For this review, take the finished solid that the model builds, in its own axes (mm). A direction names the side the tool comes from. Give positions to 0.01 mm unless a question says otherwise; leave off trailing zeros. Write each loop counter-clockwise with the first axis right and the second up, starting at its lowest first coordinate (ties: lowest second). Pieces come first, ordered by that corner, then holes. Notation, with made-up numbers: (-11, 43.25) -> (11, 43.25) arc R25 ccw to (11, 62.25) -> close; hole circle Ø9 at (24.25, 6.25). An arc over 180 degrees is marked (long way). Return JSON: item names as keys, results as strings.
from build123d import *

# Parameters (mm, degrees)
CROQUIS1_W               = 40.7
CROQUIS1_H               = 38
SALIENTE_EXTRUIR1_DEPTH  = 10.25
CROQUIS2_W               = 7
CROQUIS2_H               = 2.4
SALIENTE_EXTRUIR2_DEPTH  = 18.5
SALIENTE_EXTRUIR3_DEPTH  = 0.5
CORTAR_EXTRUIR1_DEPTH    = 2.4
SALIENTE_EXTRUIR4_DEPTH  = 2
CORTAR_EXTRUIR3_START    = -18.5
CORTAR_EXTRUIR3_DEPTH    = 18.5
CROQUIS10_R              = 7
SALIENTE_EXTRUIR5_DEPTH  = 0.75
CROQUIS11_R              = 5.5
SALIENTE_EXTRUIR6_DEPTH  = 1
CROQUIS12_R              = 3
SALIENTE_EXTRUIR7_DEPTH  = 5
CHAFL_N2_SIZE            = 0.5
CHAFL_N2_OF_MIRROR1_SIZE = 0.5


with BuildPart() as part:
    # Croquis1 → Saliente-Extruir1 (new body, symmetric)
    with BuildSketch(Plane.XY):
        Rectangle(CROQUIS1_W, CROQUIS1_H)
    extrude(amount=SALIENTE_EXTRUIR1_DEPTH, both=True)

    # Croquis2 → Saliente-Extruir2 (add)
    with BuildSketch(Plane.XY.offset(9.25)):
        with Locations((-23.85, 10.2)):
            Rectangle(CROQUIS2_W, CROQUIS2_H)
        with Locations((23.85, 10.2)):
            Rectangle(CROQUIS2_W, CROQUIS2_H)
    extrude(amount=-SALIENTE_EXTRUIR2_DEPTH)

    # Croquis3 → Saliente-Extruir3 (add, symmetric)
    with BuildSketch(Plane.XY):
        Polygon((-20.35, 12.4), (-20.35, 11.4), (-27.35, 11.4), align=None)
        Polygon((20.35, 12.4), (27.35, 11.4), (20.35, 11.4), align=None)
    extrude(amount=SALIENTE_EXTRUIR3_DEPTH, both=True)

    # Croquis4 → Cortar-Extruir1 (cut)
    with BuildSketch(Plane(origin=(0, 11.4, 0), x_dir=(1, 0, 0), z_dir=(0, 1, 0))):
        with BuildLine():
            Line((-27.35, 6.5), (-26.177050983, 6.5))
            ThreePointArc((-26.177050983, 6.5), (-22.25, 5), (-26.177050983, 3.5))
            Line((-26.177050983, 3.5), (-27.35, 3.5))
            Line((-27.35, 3.5), (-27.35, 6.5))
        make_face()
        with BuildLine():
            Line((-27.35, -3.5), (-26.177050983, -3.5))
            ThreePointArc((-26.177050983, -3.5), (-22.25, -5), (-26.177050983, -6.5))
            Line((-26.177050983, -6.5), (-27.35, -6.5))
            Line((-27.35, -6.5), (-27.35, -3.5))
        make_face()
        with BuildLine():
            Line((26.177050983, -6.5), (27.35, -6.5))
            Line((27.35, -6.5), (27.35, -3.5))
            Line((27.35, -3.5), (26.177050983, -3.5))
            ThreePointArc((26.177050983, -3.5), (22.25, -5), (26.177050983, -6.5))
        make_face()
        with BuildLine():
            Line((27.35, 3.5), (26.177050983, 3.5))
            ThreePointArc((26.177050983, 3.5), (22.25, 5), (26.177050983, 6.5))
            Line((26.177050983, 6.5), (27.35, 6.5))
            Line((27.35, 6.5), (27.35, 3.5))
        make_face()
    extrude(amount=-CORTAR_EXTRUIR1_DEPTH, mode=Mode.SUBTRACT)

    # Croquis6 → Saliente-Extruir4 (add)
    with BuildSketch(Plane(origin=(0, 19, 0), x_dir=(1, 0, 0), z_dir=(0, 1, 0))):
        with BuildLine():
            Line((10.1, 9.25), (-19.35, 9.25))
            Line((-19.35, 9.25), (-19.35, -9.25))
            Line((-19.35, -9.25), (10.1, -9.25))
            ThreePointArc((10.1, -9.25), (19.35, 0), (10.1, 9.25))
        make_face()
    saliente_extruir4 = extrude(amount=SALIENTE_EXTRUIR4_DEPTH)

    # Croquis9 → Cortar-Extruir3 (cut)
    with BuildSketch(Plane.XY.offset(9.25).offset(CORTAR_EXTRUIR3_START)):
        Polygon((-19.35, 21), (-19.35, 20), (-15.35, 20), (-14.35, 21), align=None)
    cortar_extruir3 = extrude(amount=CORTAR_EXTRUIR3_DEPTH, mode=Mode.SUBTRACT)

    # Croquis10 → Saliente-Extruir5 (add)
    with BuildSketch(Plane(origin=(0, 21, 0), x_dir=(1, 0, 0), z_dir=(0, 1, 0))):
        with Locations((10.1, 0)):
            Circle(CROQUIS10_R)
    saliente_extruir5 = extrude(amount=SALIENTE_EXTRUIR5_DEPTH)

    # Croquis11 → Saliente-Extruir6 (add)
    with BuildSketch(Plane(origin=(0, 21.75, 0), x_dir=(1, 0, 0), z_dir=(0, 1, 0))):
        with Locations((10.1, 0)):
            Circle(CROQUIS11_R)
    saliente_extruir6 = extrude(amount=SALIENTE_EXTRUIR6_DEPTH)

    # Croquis12 → Saliente-Extruir7 (add)
    with BuildSketch(Plane(origin=(0, 22.75, 0), x_dir=(1, 0, 0), z_dir=(0, 1, 0))):
        with Locations((10.1, 0)):
            Circle(CROQUIS12_R)
    saliente_extruir7 = extrude(amount=SALIENTE_EXTRUIR7_DEPTH)

    # Chaflán2
    chafl_n2_edges = [part.edges().sort_by_distance(p)[0] for p in [
        (19.35, 21, 0),
        (-2.125, 21, -9.25),
        (-2.125, 21, 9.25),
        (7.1, 27.75, 0),
    ]]
    chamfer(chafl_n2_edges, length=CHAFL_N2_SIZE)

    # Croquis13 → Cortar-Revolución1 (revolve, cut)
    with BuildSketch(Plane.XY):
        Polygon((7.1, 23.25), (7.1, 22.75), (7.6, 22.75), align=None)
    revolve(axis=Axis((10.1, 27.75, 0), (0, -1, 0)), mode=Mode.SUBTRACT)

    # Mirror1: Saliente-Extruir4, Cortar-Extruir3, Saliente-Extruir5, Saliente-Extruir6, Saliente-Extruir7 across plane
    add(saliente_extruir4.mirror(Plane.ZX))
    add(cortar_extruir3.mirror(Plane.ZX), mode=Mode.SUBTRACT)
    add(saliente_extruir5.mirror(Plane.ZX))
    add(saliente_extruir6.mirror(Plane.ZX))
    add(saliente_extruir7.mirror(Plane.ZX))

    # Chaflán2 of Mirror1
    chafl_n2_of_mirror1_edges = [part.edges().sort_by_distance(p)[0] for p in [
        (19.35, -21, 0),
        (-2.125, -21, -9.25),
        (-2.125, -21, 9.25),
        (7.1, -27.75, 0),
    ]]
    chamfer(chafl_n2_of_mirror1_edges, length=CHAFL_N2_OF_MIRROR1_SIZE)


solid = part.part
1. For pin 1 (2.5 mm diameter, centred on x = 23, y = 10, fed in from -Z); pin 2 (6 mm diameter, centred on y = -17.5, z = -5, fed in from -X); pin 3 (2 mm diameter, centred on x = -25.5, z = -1, fed in from -Y); pin 4 (10 mm diameter, centred on x = 20.5, y = 17, fed in from -Z), all flat-tipped, find the tip position at first contact; note any pin that passes through.
Results found:
{"pin 1": "stops at z = -9.25", "pin 2": "stops at x = -20.35", "pin 3": "stops at y = 9", "pin 4": "stops at z = -10.25"}
2. Add section C-C, the plane y = -5.5. State the section outline as (x, z) points, plus the area to 3 significant figures.
Results found:
{"outline": "(-20.35, -10.25) -> (20.35, -10.25) -> (20.35, 10.25) -> (-20.35, 10.25) -> close", "area": "834 mm²"}
3. The part is to be moulded in two halves that separate along Z. For faces 1 (the flat face through (0, 0, -10.25)), 2 (the cylindrical face through (19.348, 19.74, 0.203)), 3 (the flat face through (-27.35, 10, 8)), 4 (the cylindrical face through (-22.25, 10.22, -5.08)), say which applies: +Z half, -Z half, draft (parallel to the pull), parting line (faces both ways), or undercut.
Results found:
{"face 1": "-Z half", "face 2": "parting line", "face 3": "draft", "face 4": "undercut"}
4. To check wall thickness, follow probe 1 along Z at (x, y) = (-24.5, 9.55); probe 2 along X at (y, z) = (-18.5, 7.5); probe 3 along Y at (x, z) = (11.5, -3.75). State the ranges of each line that lie inside material, in increasing order.
Results found:
{"probe 1": "z = -9.25 to -7.25, -2.75 to 2.75, 7.25 to 9.25", "probe 2": "x = -20.35 to 20.35", "probe 3": "y = -22.75 to 22.75"}
5. Add section A-A, the plane x = 24.5. State the section outline as (y, z) points, plus the area to 3 significant figures.
Results found:
{"outline": "(9, -9.25) -> (11.4, -9.25) -> (11.4, -7.25) -> (9, -7.25) -> close; (9, -2.75) -> (11.4, -2.75) -> (11.4, -0.5) -> (11.81, -0.5) -> (11.81, 0.5) -> (11.4, 0.5) -> (11.4, 2.75) -> (9, 2.75) -> close; (9, 7.25) -> (11.4, 7.25) -> (11.4, 9.25) -> (9, 9.25) -> close", "area": "23.2 mm²"}
6. For faces 5 (the cylindrical face through (7.1, -25, -0.1)), 6 (the flat face through (-22, 11.4, 4)), 7 (the flat face through (24, 10, -9.25)), 8 (the flat face through (-5, 20, 9.25)), list the 3-axis set-ups (+Z, -Z, +X, -X, +Y, -Y) from which the entire face can be reached by the end or side of a thin tool; tool diameter is ignored.
Results found:
{"face 5": "-Y", "face 6": "+Z, -X, +Y", "face 7": "-Z, +X, +Y, -Y", "face 8": "+Z, +X, -X, +Y"}
7. Add section B-B, the plane x = 1. State the section outline as (y, z) points, plus the area to 4 significant figures.
Results found:
{"outline": "(-21, -8.75) -> (-20.5, -9.25) -> (-19, -9.25) -> (-19, -10.25) -> (19, -10.25) -> (19, -9.25) -> (20.5, -9.25) -> (21, -8.75) -> (21, 8.75) -> (20.5, 9.25) -> (19, 9.25) -> (19, 10.25) -> (-19, 10.25) -> (-19, 9.25) -> (-20.5, 9.25) -> (-21, 8.75) -> close", "area": "852.5 mm²"}
